For this review, take the finished solid that the model builds, in its own axes (mm). Face numbers are marked on the shaded views. A direction names the side the tool comes from. Round coordinates to 2 decimals unless told otherwise and drop trailing zeros. Order: outer loops, then holes, each group sorted by start corner. A loop starts at its lowest first (then second) coordinate and runs counter-clockwise, first axis right, second up. Notation, with made-up numbers: (30, -32) -> (44, -32) arc R9 cw to (44, -16) -> close; hole circle Ø10 at (57, 39.5). An arc over 180 degrees is marked (long way). Answer in a Markdown table with one row per item.
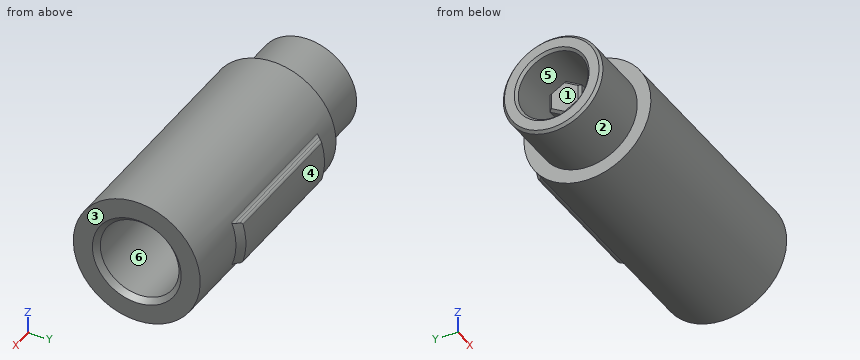
```python
from build123d import *

# Parameters (mm, degrees)
SKETCH_1_R          = 5
EXTRUDE_1_DEPTH     = 19
SKETCH_3_R          = 3.1
CUT_EXTRUDE_1_DEPTH = 17
EXTRUDE_2_DEPTH     = 12
SKETCH_8_R          = 3.925
EXTRUDE_4_DEPTH     = 5
SKETCH_9_R          = 2.75
CUT_EXTRUDE_2_DEPTH = 5
EXTRUDE_5_DEPTH     = 3.2
FILLET_1_R          = 0.2
CHAMFER_1_SIZE      = 0.5
CHAMFER_2_SIZE      = 0.4
CHAMFER_3_SIZE      = 0.2


with BuildPart() as part:
    # 草图1 → 凸台-拉伸1 (new body)
    with BuildSketch(Plane(origin=(0, 0, 0), x_dir=(0, 0, -1), z_dir=(1, 0, 0))):
        Circle(SKETCH_1_R)
    extrude(amount=EXTRUDE_1_DEPTH)

    # 草图3 → 切除-拉伸1 (cut)
    with BuildSketch(Plane(origin=(19, 0, 0), x_dir=(0, 0, -1), z_dir=(1, 0, 0))):
        Circle(SKETCH_3_R)
    extrude(amount=-CUT_EXTRUDE_1_DEPTH, mode=Mode.SUBTRACT)

    # 草图5 → 凸台-拉伸2 (add)
    with BuildSketch(Plane(origin=(2, 0, 0), x_dir=(0, 0, -1), z_dir=(1, 0, 0))):
        with BuildLine():
            Line((-1.688194302, 2.6), (1.688194302, 2.6))
            Line((1.688194302, 2.6), (1.688194302, 5.234500931))
            ThreePointArc((1.688194302, 5.234500931), (0, 5.5), (-1.688194302, 5.234500931))
            Line((-1.688194302, 5.234500931), (-1.688194302, 2.6))
        make_face()
    extrude(amount=EXTRUDE_2_DEPTH)

    # 草图8 → 凸台-拉伸4 (add)
    with BuildSketch(Plane.ZY):
        Circle(SKETCH_8_R)
    extrude(amount=EXTRUDE_4_DEPTH)

    # 草图9 → 切除-拉伸2 (cut)
    with BuildSketch(Plane.ZY.offset(5)):
        Circle(SKETCH_9_R)
    extrude(amount=-CUT_EXTRUDE_2_DEPTH, mode=Mode.SUBTRACT)

    # 草图10 → 凸台-拉伸5 (add)
    with BuildSketch(Plane.ZY):
        Polygon((0.721687836, 1.25), (-0.721687836, 1.25), (-1.443375673, 0), (-0.721687836, -1.25), (0.721687836, -1.25), (1.443375673, 0), align=None)
    extrude(amount=EXTRUDE_5_DEPTH)

    # 圆角1
    fillet_1_edges = [part.edges().sort_by_distance(p)[0] for p in [
        (8, 4.70637865, 1.688194302),
        (8, 5.234500931, 1.688194302),
        (8, 4.70637865, -1.688194302),
        (8, 5.234500931, -1.688194302),
    ]]
    fillet(fillet_1_edges, radius=FILLET_1_R)

    # 倒角1
    # the kernel refuses this chamfer: 0.5 mm, written as the material it takes off along each edge
    with BuildSketch(Plane(origin=(14, 0, 0), x_dir=(0, 0.8686030413593419, -0.4955085837211114), z_dir=(0, -0.4955085837211114, -0.8686030413593419))) as chamfer_1_piece_1:
        Polygon((5.5, -CHAMFER_1_SIZE), (5.5 - CHAMFER_1_SIZE, 0), (5.5, 0), align=None)
    revolve(axis=Axis((14, 0, 0), (1, 0, 0)), revolution_arc=59.40658503, mode=Mode.SUBTRACT)
    with BuildSketch(Plane(origin=(2, 0, 0), x_dir=(0, 0.8686030413593415, -0.4955085837211117), z_dir=(0, -0.4955085837211117, -0.8686030413593415))) as chamfer_1_piece_2:
        Polygon((5.5 - CHAMFER_1_SIZE, 0), (5.5, CHAMFER_1_SIZE), (5.5, 0), align=None)
    revolve(axis=Axis((2, 0, 0), (1, 0, 0)), revolution_arc=59.40658503, mode=Mode.SUBTRACT)
    with BuildSketch(Plane(origin=(14, 2.6, 2.974035796), x_dir=(0.027495876610585623, 0.9996219169112968, 0), z_dir=(0, 0, -1))) as chamfer_1_piece_3_section:
        Polygon((CHAMFER_1_SIZE * 0.999621916911, -CHAMFER_1_SIZE * 0.0274958766106), (-CHAMFER_1_SIZE * 0.0274958766106, -CHAMFER_1_SIZE * 0.999621916911), (0, 0), align=None)
    chamfer_1_piece_3 = extrude(amount=5.948071591, mode=Mode.PRIVATE)
    chamfer_1_piece_3 = chamfer_1_piece_3 & Plane(origin=(13.821912141, 0, 0), x_dir=(0, 0, -1), z_dir=(1, 0, 0)) * Cylinder(3.1, 14, mode=Mode.PRIVATE)
    add(chamfer_1_piece_3, mode=Mode.SUBTRACT)

    # 倒角2
    chamfer_2_edges = [part.edges().sort_by_distance(p)[0] for p in [
        (19, 0, 3.1),
    ]]
    chamfer(chamfer_2_edges, length=CHAMFER_2_SIZE)

    # 倒角3
    chamfer_3_edges = [part.edges().sort_by_distance(p)[0] for p in [
        (-5, 0, -3.925),
        (-5, 0, -2.75),
        (-3.2, 0.625, 1.082531755),
        (-3.2, 1.25, 0),
        (-3.2, 0.625, -1.082531755),
        (-3.2, -0.625, -1.082531755),
        (-3.2, -1.25, 0),
        (-3.2, -0.625, 1.082531755),
    ]]
    chamfer(chamfer_3_edges, length=CHAMFER_3_SIZE)


solid = part.part
```
Q1. Tool access review of the marked faces 4, 5 and 6: name each direction out of +Z, -Z, +X, -X, +Y, -Y from which nothing blocks a thin tool from reaching the whole face with its end or side.
Answer key:
| item | result |
|---|---|
| face 4 | +X, -X, +Y |
| face 5 | -X |
| face 6 | +X |
Q2. Take a section at A-A, the plane x = -0.5. Write out the cut boundary in (y, z) (3 decimals).
Answer key:
| item | result |
|---|---|
| outline | circle Ø7.85 at (0, 0); (-1.25, -0.722) -> (0, -1.443) -> (1.25, -0.722) -> (1.25, 0.722) -> (0, 1.443) -> (-1.25, 0.722) -> close; hole circle Ø5.5 at (0, 0) |
Q3. Clearance check with flat-ended pins moving along their axes: pin 1 Ø2 at (x, z) = (0, 4) entering from +Y; pin 2 Ø0.7 at (x, z) = (-1.5, 0) entering from +Y (3 decimals); pin 3 Ø6 at (y, z) = (1, 0) entering from +X; pin 4 Ø1.6 at (y, z) = (0.5, 1) entering from -X. State where each tip first meets the part, or that it passes through.
Answer key:
| item | result |
|---|---|
| pin 1 | stops at y = 4 |
| pin 2 | stops at y = 3.925 |
| pin 3 | stops at x = 19 |
| pin 4 | stops at x = -3.2 |
Q4. To check wall thickness, follow probe 1 along Y at (x, z) = (2.75, 0); probe 2 along Y at (x, z) = (-2, 0.75); probe 3 along X at (y, z) = (3.5, 3). State the ranges of each line that lie inside material, in increasing order.
Answer key:
| item | result |
|---|---|
| probe 1 | y = -5 to -3.1, 2.6 to 5.5 |
| probe 2 | y = -3.85 to -2.65, -1.2 to 1.2, 2.65 to 3.85 |
| probe 3 | x = 0 to 19 |
Q5. Take a section at D-D, the plane y = -4.25. Write out the cut boundary in (x, z), then the cut area to 3 significant figures.
Answer key:
| item | result |
|---|---|
| outline | (0, -2.63) -> (19, -2.63) -> (19, 2.63) -> (0, 2.63) -> close |
| area | 100 mm^2 |
Q6. The part is to be moulded in two halves that separate along Y. For the marked faces 1, 2 and 3, say which applies: +Y half, -Y half, draft (parallel to the pull), parting line (faces both ways), or undercut.
Answer key:
| item | result |
|---|---|
| face 1 | undercut |
| face 2 | parting line |
| face 3 | draft |
Q7. Take a section at C-C, the plane x = 12.5. Write out the cut boundary in (y, z).
Answer key:
| item | result |
|---|---|
| outline | (4.66, -1.82) arc R0.2 cw to (4.85, -1.69) -> (5.09, -1.69) arc R0.2 ccw to (5.28, -1.54) arc R5.5 ccw to (5.28, 1.54) arc R0.2 ccw to (5.09, 1.69) -> (4.85, 1.69) arc R0.2 cw to (4.66, 1.82) arc R5 ccw (long way) to start; hole (2.6, -1.69) -> (2.6, 1.69) arc R3.1 ccw (long way) to start |
